```python
from build123d import *

# Parameters (mm, degrees)
SKETCH1_W                      = 221.6
SKETCH1_H                      = 94
BOSS_EXTRUDE1_DEPTH            = 6.35
CUT_EXTRUDE1_REACH             = 122.524
SKETCH3_R                      = 4
CHAMFER1_SIZE                  = 1
SKETCH6_R                      = 5
CUT_EXTRUDE2_DEPTH             = 121.523700989
CHAMFER2_SIZE                  = 4.35
CHAMFER2_SIZE2                 = 0.22797384
CHAMFER3_SIZE                  = 4.35
CHAMFER3_SIZE2                 = 0.22797384
SKETCH11_R                     = 12.7
CUT_EXTRUDE3_DEPTH             = 121.523700994
M8_CLEARANCE_HOLE1_AT_2_COUNT  = 2
M8_CLEARANCE_HOLE1_AT_2_PITCH  = 74
M8_CLEARANCE_HOLE1_AT_3_COUNT  = 2
M8_CLEARANCE_HOLE1_AT_3_PITCH  = 201.6
M8_CLEARANCE_HOLE1_AT_4_COUNT  = 2
M8_CLEARANCE_HOLE1_AT_4_PITCH  = 214.752322455
M8_CLEARANCE_HOLE1_AT_5_COUNT  = 2
M8_CLEARANCE_HOLE1_AT_5_PITCH  = 100.8
M8_CLEARANCE_HOLE1_AT_6_COUNT  = 2
M8_CLEARANCE_HOLE1_AT_6_PITCH  = 125.046551332
F_8_0MM_DOWEL_HOLE1_AT_2_COUNT = 2
F_8_0MM_DOWEL_HOLE1_AT_2_PITCH = 74
F_8_0MM_DOWEL_HOLE1_AT_3_COUNT = 2
F_8_0MM_DOWEL_HOLE1_AT_3_PITCH = 167.6
F_8_0MM_DOWEL_HOLE1_AT_4_COUNT = 2
F_8_0MM_DOWEL_HOLE1_AT_4_PITCH = 183.209606735
M6_TAPPED_HOLE1_AT_2_COUNT     = 2
M6_TAPPED_HOLE1_AT_2_PITCH     = 38.1


with BuildPart() as part:
    # Sketch1 → Boss-Extrude1 (new body)
    with BuildSketch(Plane(origin=(0, 0, 0), x_dir=(1, 0, 0), z_dir=(0, 1, 0))):
        Rectangle(SKETCH1_W, SKETCH1_H)
    extrude(amount=-BOSS_EXTRUDE1_DEPTH)

    # Sketch3 → Cut-Extrude1 (cut, up to next)
    with BuildSketch(Plane(origin=(0, 0, 0), x_dir=(1, 0, 0), z_dir=(0, 1, 0)), mode=Mode.PRIVATE) as cut_extrude1_sk1:
        with Locations(Location((-53.025, 0, 0), (0, 0, 270))):
            Circle(SKETCH3_R)
    cut_extrude1_tool1 = extrude(cut_extrude1_sk1.sketch, amount=-CUT_EXTRUDE1_REACH, mode=Mode.PRIVATE) & part.part
    add(cut_extrude1_tool1.solids().sort_by_distance((-53.025, 0, 0))[0], mode=Mode.SUBTRACT)

    # Chamfer1
    chamfer1_edges = [part.edges().sort_by_distance(p)[0] for p in [
        (-110.8, -6.35, 0),
        (0, -6.35, 47),
        (110.8, -6.35, 0),
        (0, 0, 47),
        (-110.8, 0, 0),
        (0, 0, -47),
        (110.8, 0, 0),
        (110.8, -3.175, 47),
        (-110.8, -3.175, 47),
        (-110.8, -3.175, -47),
        (0, -6.35, -47),
    ]]
    chamfer(chamfer1_edges, length=CHAMFER1_SIZE)

    # Sketch6 → Cut-Extrude2 (cut, through all)
    with BuildSketch(Plane(origin=(0, 0, 0), x_dir=(1, 0, 0), z_dir=(0, 1, 0))):
        with Locations(Location((73.8, 0, 0), (0, 0, 270))):
            Circle(SKETCH6_R)
        with Locations(Location((35.8, 0, 0), (0, 0, 270))):
            Circle(SKETCH6_R)
        with BuildLine():
            Line((-33.8, 15), (4.2, 15))
            ThreePointArc((4.2, 15), (19.2, 0), (4.2, -15))
            Line((4.2, -15), (-33.8, -15))
            ThreePointArc((-33.8, -15), (-48.8, 0), (-33.8, 15))
        make_face()
    extrude(amount=-CUT_EXTRUDE2_DEPTH, mode=Mode.SUBTRACT)

    # Cut-Sweep1: sweep along a path in Sketch2
    with BuildLine(Plane(origin=(0, 0, 0), x_dir=(1, 0, 0), z_dir=(0, 1, 0))) as cut_sweep1_path:
        Line((-33.8, 15), (4.2, 15))
        ThreePointArc((4.2, 15), (19.2, 0), (4.2, -15))
        Line((4.2, -15), (-33.8, -15))
        ThreePointArc((-33.8, -15), (-48.8, 0), (-33.8, 15))
    # Sketch10 → Cut-Sweep1 (sweep, cut)
    with BuildSketch(Plane(origin=(-33.8, 0, 0), x_dir=(0, 0, -1), z_dir=(1, 0, 0))):
        Polygon((15, -4.35), (15.22797384, 0), (15, 0), align=None)
    sweep(path=cut_sweep1_path.line, mode=Mode.SUBTRACT)

    # Chamfer2
    chamfer2_edges = [part.edges().sort_by_distance(p)[0] for p in [
        (35.8, 0, -5),
    ]]
    chamfer2_side = [part.faces().sort_by_distance(p)[0] for p in [
        (35.8, -3.175, -5),
    ]]
    chamfer(chamfer2_edges, length=CHAMFER2_SIZE, length2=CHAMFER2_SIZE2, reference=chamfer2_side[0])

    # Chamfer3
    chamfer3_edges = [part.edges().sort_by_distance(p)[0] for p in [
        (73.8, 0, -5),
    ]]
    chamfer3_side = [part.faces().sort_by_distance(p)[0] for p in [
        (73.8, -3.175, -5),
    ]]
    chamfer(chamfer3_edges, length=CHAMFER3_SIZE, length2=CHAMFER3_SIZE2, reference=chamfer3_side[0])

    # Sketch11 → Cut-Extrude3 (cut, through all)
    with BuildSketch(Plane(origin=(0, 0, 0), x_dir=(1, 0, 0), z_dir=(0, 1, 0))):
        with Locations(Location((-87.95, 0, 0), (0, 0, 270))):
            Circle(SKETCH11_R)
    extrude(amount=-CUT_EXTRUDE3_DEPTH, mode=Mode.SUBTRACT)

    # Sketch13 → M8 Clearance Hole1 (revolve, cut)
    with BuildSketch(Plane(origin=(-100.8, 0, -37), x_dir=(0, 0, 1), z_dir=(1, 0, 0))):
        Polygon((0, 0), (0, 6.35), (4.525, 6.35), (4.5, 6.325), (4.5, 0.025), (4.525, 0), align=None)
    m8_clearance_hole1 = revolve(axis=Axis((-100.8, 6.35, -37), (0, -1, 0)), mode=Mode.SUBTRACT)

    # M8 Clearance Hole1 at 2: M8 Clearance Hole1 ×2
    with Locations(*[(0, 0, i * M8_CLEARANCE_HOLE1_AT_2_PITCH) for i in range(1, M8_CLEARANCE_HOLE1_AT_2_COUNT)]):
        add(m8_clearance_hole1, mode=Mode.SUBTRACT)

    # M8 Clearance Hole1 at 3: M8 Clearance Hole1 ×2
    with Locations(*[(i * M8_CLEARANCE_HOLE1_AT_3_PITCH, 0, 0) for i in range(1, M8_CLEARANCE_HOLE1_AT_3_COUNT)]):
        add(m8_clearance_hole1, mode=Mode.SUBTRACT)

    # M8 Clearance Hole1 at 4: M8 Clearance Hole1 ×2
    with Locations(*[Vector(0.9387558546280332, 0, 0.34458300219481375) * (i * M8_CLEARANCE_HOLE1_AT_4_PITCH) for i in range(1, M8_CLEARANCE_HOLE1_AT_4_COUNT)]):
        add(m8_clearance_hole1, mode=Mode.SUBTRACT)

    # M8 Clearance Hole1 at 5: M8 Clearance Hole1 ×2
    with Locations(*[(i * M8_CLEARANCE_HOLE1_AT_5_PITCH, 0, 0) for i in range(1, M8_CLEARANCE_HOLE1_AT_5_COUNT)]):
        add(m8_clearance_hole1, mode=Mode.SUBTRACT)

    # M8 Clearance Hole1 at 6: M8 Clearance Hole1 ×2
    with Locations(*[Vector(0.8060997998454218, 0, 0.591779614965885) * (i * M8_CLEARANCE_HOLE1_AT_6_PITCH) for i in range(1, M8_CLEARANCE_HOLE1_AT_6_COUNT)]):
        add(m8_clearance_hole1, mode=Mode.SUBTRACT)

    # Sketch15 → Ø8.0mm Dowel Hole1 (revolve, cut)
    with BuildSketch(Plane(origin=(-83.8, 0, -37), x_dir=(0, 0, 1), z_dir=(1, 0, 0))):
        Polygon((0, 0), (0, 6.35), (4.025, 6.35), (4, 6.325), (4, 0.025), (4.025, 0), align=None)
    f_8_0mm_dowel_hole1 = revolve(axis=Axis((-83.8, 6.35, -37), (0, -1, 0)), mode=Mode.SUBTRACT)

    # Ø8.0mm Dowel Hole1 at 2: Ø8.0mm Dowel Hole1 ×2
    with Locations(*[(0, 0, i * F_8_0MM_DOWEL_HOLE1_AT_2_PITCH) for i in range(1, F_8_0MM_DOWEL_HOLE1_AT_2_COUNT)]):
        add(f_8_0mm_dowel_hole1, mode=Mode.SUBTRACT)

    # Ø8.0mm Dowel Hole1 at 3: Ø8.0mm Dowel Hole1 ×2
    with Locations(*[(i * F_8_0MM_DOWEL_HOLE1_AT_3_PITCH, 0, 0) for i in range(1, F_8_0MM_DOWEL_HOLE1_AT_3_COUNT)]):
        add(f_8_0mm_dowel_hole1, mode=Mode.SUBTRACT)

    # Ø8.0mm Dowel Hole1 at 4: Ø8.0mm Dowel Hole1 ×2
    with Locations(*[Vector(0.9147991908656035, 0, 0.40390895062085114) * (i * F_8_0MM_DOWEL_HOLE1_AT_4_PITCH) for i in range(1, F_8_0MM_DOWEL_HOLE1_AT_4_COUNT)]):
        add(f_8_0mm_dowel_hole1, mode=Mode.SUBTRACT)

    # Sketch17 → M6 Tapped Hole1 (revolve, cut)
    with BuildSketch(Plane(origin=(-87.95, 0, -19.05), x_dir=(0, 0, 1), z_dir=(1, 0, 0))):
        Polygon((0, 0), (0, 6.35), (3.025, 6.35), (2.5, 5.825), (2.5, 0.525), (3.025, 0), align=None)
    m6_tapped_hole1 = revolve(axis=Axis((-87.95, 6.35, -19.05), (0, -1, 0)), mode=Mode.SUBTRACT)

    # M6 Tapped Hole1 at 2: M6 Tapped Hole1 ×2
    with Locations(*[(0, 0, i * M6_TAPPED_HOLE1_AT_2_PITCH) for i in range(1, M6_TAPPED_HOLE1_AT_2_COUNT)]):
        add(m6_tapped_hole1, mode=Mode.SUBTRACT)


solid = part.part
```
Can you work these out from the model? Positions are in its coordinate system, mm. Give positions to 0.01 mm unless a question says otherwise; leave off trailing zeros. Loops run counter-clockwise (first coordinate to the right, second up) from the corner with the lowest first, then second, coordinate; pieces in that order, holes last. Notation, with made-up numbers: M 70.5,65.5 L 123.5,65.5 A28 ccw 123.5,84.5 Z; hole C 19,85 d2. An arc over 180 degrees is marked long. Answer in a Markdown table with one row per item.
1. Suppose I cut it at C-C on y = -2.25. Count the separate pieces of the cut face and the enclosed holes in it, plus the area to 3 significant figures.
Taken from the geometry:
| item | result |
|---|---|
| separate pieces | 1 |
| enclosed holes | 17 |
| area | 17,600 mm² |
2. For pin 1 Ø10.5 at (x, z) = (83.8, 37) entering from -Y; pin 2 Ø8 at (x, z) = (0, -37) entering from +Y, each with a flat end and sliding along its axis, tell me the tip position at first contact or that it passes through.
Taken from the geometry:
| item | result |
|---|---|
| pin 1 | stops at y = -6.35 |
| pin 2 | passes through |
3. Thinking about a two-plate mould opening in X: for faces 1 (the flat face through (-2, -6.35, -21)), 2 (the cylindrical face through (-96.81, -3.13, -34.92)), which applies, released by +X, released by -X, zero draft, split by the parting line, or undercut?
Taken from the geometry:
| item | result |
|---|---|
| face 1 | zero draft |
| face 2 | undercut |
4. Suppose I cut it at A-A on x = 83.8. Write out the boundary of the cut face in (y, z) (3 decimals).
Taken from the geometry:
| item | result |
|---|---|
| outline | M -6.35,-46 L -5.35,-47 L -1,-47 L 0,-46 L 0,-41.025 L -0.025,-41 L -6.325,-41 L -6.35,-41.025 Z; M -6.35,-32.975 L -6.325,-33 L -0.025,-33 L 0,-32.975 L 0,32.975 L -0.025,33 L -6.325,33 L -6.35,32.975 Z; M -6.35,41.025 L -6.325,41 L -0.025,41 L 0,41.025 L 0,46 L -1,47 L -5.35,47 L -6.35,46 Z |
5. If I drill on line 1 along Z through (x, y) = (100.8, -2.5); line 2 along X through (y, z) = (-2.5, 37); line 3 along X through (y, z) = (-4.85, 0) (3 decimals), over which ranges is the centre line in solid material (lowest first)?
Taken from the geometry:
| item | result |
|---|---|
| line 1 | z = -47 to -41.5, -32.5 to 32.5, 41.5 to 47 |
| line 2 | x = -110.8 to -105.3, -96.3 to -87.8, -79.8 to -4.5, 4.5 to 79.8, 87.8 to 96.3, 105.3 to 110.8 |
| line 3 | x = -110.8 to -100.65, -75.25 to -57.025, -49.025 to -48.8, 19.2 to 30.8, 40.8 to 68.8, 78.8 to 110.8 |
6. Suppose I cut it at B-B on z = -19.05. Write out the boundary of the cut face in (x, y) (3 decimals).
Taken from the geometry:
| item | result |
|---|---|
| outline | M -110.8,-5.35 L -109.8,-6.35 L -90.975,-6.35 L -90.45,-5.825 L -90.45,-0.525 L -90.975,0 L -109.8,0 L -110.8,-1 Z; M -85.45,-5.825 L -84.925,-6.35 L 109.8,-6.35 L 110.8,-5.35 L 110.8,-1 L 109.8,0 L -84.925,0 L -85.45,-0.525 Z |
7. Suppose I cut it at D-D on x = -8. Write out the boundary of the cut face in (y, z), plus the area to 3 significant figures.
Taken from the geometry:
| item | result |
|---|---|
| outline | M -6.35,-46 L -5.35,-47 L -1,-47 L 0,-46 L 0,-15.23 L -4.35,-15 L -6.35,-15 Z; M -6.35,15 L -4.35,15 L 0,15.23 L 0,46 L -1,47 L -5.35,47 L -6.35,46 Z |
| area | 403 mm² |
